For this review, take the finished solid that the model builds, in its own axes (mm). A direction names the side the tool comes from. Round coordinates to 2 decimals unless told otherwise and drop trailing zeros. Loops run counter-clockwise (first coordinate to the right, second up) from the corner with the lowest first, then second, coordinate; pieces in that order, holes last.
```python
from build123d import *

# Parameters (mm, degrees)
SKETCH1_W           = 80
SKETCH1_H           = 80
BOSS_EXTRUDE1_DEPTH = 15
BOSS_EXTRUDE1_DRAFT = -5
SKETCH2_W           = 13.5
SKETCH2_H           = 72
SKETCH2_W_2         = 72
SKETCH2_H_2         = 13.5
CUT_EXTRUDE1_DEPTH  = 10
CUT_EXTRUDE1_TAPER  = 5
SKETCH3_R           = 27.5
BOSS_EXTRUDE2_DEPTH = 10
SKETCH4_W           = 100
SKETCH4_H           = 100
BOSS_EXTRUDE3_DEPTH = 20
SKETCH5_R           = 2.5
BOSS_EXTRUDE4_DEPTH = 10
CIRPATTERN1_COUNT   = 4
SKETCH6_R           = 10
CUT_EXTRUDE2_DEPTH  = 25
CUT_EXTRUDE2_DRAFT  = -20


with BuildPart() as part:
    # Sketch1 → Boss-Extrude1 (with draft: the straight prism first)
    with BuildSketch(Plane(origin=(0, 0, 0), x_dir=(1, 0, 0), z_dir=(0, 1, 0))):
        Rectangle(SKETCH1_W, SKETCH1_H)
    extrude(amount=BOSS_EXTRUDE1_DEPTH)
    # Boss-Extrude1: the draft: its side faces are tilted about the plane it starts from
    boss_extrude1_sides = [part.faces().sort_by_distance(p)[0] for p in [
        (0, 7.5, 40),
        (40, 7.5, 0),
        (0, 7.5, -40),
        (-40, 7.5, 0),
    ]]
    draft(boss_extrude1_sides, Plane(origin=(0, 0, 0), x_dir=(1, 0, 0), z_dir=(0, 1, 0)), BOSS_EXTRUDE1_DRAFT)

    # Sketch2 → Cut-Extrude1 (cut)
    with BuildSketch(Plane(origin=(0, 15, 0), x_dir=(1, 0, 0), z_dir=(0, 1, 0))):
        Rectangle(SKETCH2_W, SKETCH2_H)
        Rectangle(SKETCH2_W_2, SKETCH2_H_2)
    extrude(amount=-CUT_EXTRUDE1_DEPTH, taper=CUT_EXTRUDE1_TAPER, mode=Mode.SUBTRACT)

    # Sketch3 → Boss-Extrude2 (add)
    with BuildSketch(Plane.XZ):
        with Locations(Location((0, 0, 0), (0, 0, 270))):  # turned: the seam where the file's is
            Circle(SKETCH3_R)
    extrude(amount=BOSS_EXTRUDE2_DEPTH)


with BuildPart() as body_2:
    # Sketch4 → Boss-Extrude3 (new body)
    with BuildSketch(Plane.XZ):
        Rectangle(SKETCH4_W, SKETCH4_H)
    extrude(amount=BOSS_EXTRUDE3_DEPTH)

    # Combine1: cut part
    add(part.part, mode=Mode.SUBTRACT)

    # Sketch5 → Boss-Extrude4 (add)
    with BuildSketch(Plane(origin=(0, 0, 0), x_dir=(1, 0, 0), z_dir=(0, 1, 0))):
        with Locations(Location((-45, 45, 0), (0, 0, 270))):  # turned: the seam where the file's is
            Circle(SKETCH5_R)
    boss_extrude4 = extrude(amount=BOSS_EXTRUDE4_DEPTH)

    # CirPattern1: Boss-Extrude4 ×4 about axis
    cirpattern1_axis = Axis((0, 0, 0), (0, 1, 0))
    for i in range(1, CIRPATTERN1_COUNT):
        add(boss_extrude4.rotate(cirpattern1_axis, i * 360 / CIRPATTERN1_COUNT))


with BuildPart() as cut_extrude2_tool:
    # Sketch6 → Cut-Extrude2 (with draft: the straight prism first)
    with BuildSketch(Plane.ZY.offset(50)):
        Circle(SKETCH6_R)
    extrude(amount=-CUT_EXTRUDE2_DEPTH)
    # Cut-Extrude2: the draft: its side faces are tilted about the plane it starts from
    cut_extrude2_sides = [cut_extrude2_tool.faces().sort_by_distance(p)[0] for p in [
        (-37.5, 0, -10),
    ]]
    draft(cut_extrude2_sides, Plane.ZY.offset(50), CUT_EXTRUDE2_DRAFT)


with BuildPart() as body_2_1:
    add(body_2.part)

    # Cut-Extrude2: cut by cut_extrude2_tool
    add(cut_extrude2_tool.part, mode=Mode.SUBTRACT)


solid = body_2_1.part
```
(1) Add section A-A (x = 0). Give the boundary of the cut face in (y, z), plus the area to 3 significant figures.
(2) Add section C-C (y = 7.5). Give the boundary of the cut face in (x, z).
(3) For L1, parallel to Z at x = 0, y = -7.5; L2, parallel to Y at x = -27.5, z = 12; L3, parallel to Y at x = 8.5, z = 3, list the stretches that pass through material, from the lowest coordinate up.
(4) Insertion check: pin 1 Ø8 at (x, z) = (-36.5, -2.5) entering from +Y; pin 2 Ø8 at (x, z) = (-8.5, -7.5) entering from +Y; pin 3 Ø10 at (x, y) = (-17, 6) entering from +Z. Each pin has a flat end and moves straight along its axis. Give the tip position at first contact, or say it passes through.
(5) The part is to be moulded in two halves that separate along Z. For faces 3 (the flat face through (-1, -10, -50)), 4 (the conical face through (-38.88, -5.95, -0.13)), 5 (the flat face through (-1, -10, 50)), say which applies: pulls with the +Z half, pulls with the -Z half, needs draft (parallel to the pull), parting line crosses it, or undercut.
(6) Add section B-B (z = 45). Give the boundary of the cut face in (x, y), plus the area to 3 significant figures.
(7) Add section D-D (x = 45). Give the boundary of the cut face in (y, z), plus the area to 3 significant figures.
(8) For faces 1 (the flat face through (-45, 10, -45)), 2 (the cylindrical face through (-45.96, 4.93, -42.69)), list the 3-axis set-ups (+Z, -Z, +X, -X, +Y, -Y) from which the entire face can be reached by the end or side of a thin tool; tool diameter is ignored.
Outcome:
1. outline: (-20, -50) - (0, -50) - (0, -27.5) - (-10, -27.5) - (-10, 27.5) - (0, 27.5) - (0, 50) - (-20, 50) - close
1. area: 1,450 mm2
2. outline: circle Ø5 at (-45, -45); circle Ø5 at (-45, 45); circle Ø5 at (45, -45); circle Ø5 at (45, 45)
3. L1: z = -50 to -27.5, 27.5 to 50
3. L2: y = -20 to 0
3. L3: y = -20 to -10
4. pin 1: stops at y = 0
4. pin 2: stops at y = -10
4. pin 3: passes through
5. face 3: pulls with the -Z half
5. face 4: undercut
5. face 5: pulls with the +Z half
6. outline: (-50, -20) - (50, -20) - (50, 0) - (47.5, 0) - (47.5, 10) - (42.5, 10) - (42.5, 0) - (-42.5, 0) - (-42.5, 10) - (-47.5, 10) - (-47.5, 0) - (-50, 0) - close
6. area: 2,100 mm2
7. outline: (-20, -50) - (0, -50) - (0, -47.5) - (10, -47.5) - (10, -42.5) - (0, -42.5) - (0, 42.5) - (10, 42.5) - (10, 47.5) - (0, 47.5) - (0, 50) - (-20, 50) - close
7. area: 2,100 mm2
8. face 1: +Z, -Z, +X, -X, +Y
8. face 2: +Y
